Build history of the part. All positions in model axes, mm. A direction names the side the tool comes from. Coordinates: 2 decimals unless noted, no trailing zeros. Write each loop counter-clockwise with the first axis right and the second up, starting at its lowest first coordinate (ties: lowest second). Pieces come first, ordered by that corner, then holes. Notation, with made-up numbers: (-22, 52) -> (18, 52) arc R21 cw to (18, 80) -> close; hole circle Ø11 at (25, 1.5). An arc over 180 degrees is marked (long way). Write each question's results on one line, items separated by ' | '. Start each with the question number.
Q1. Saw through at B-B on x = 124. Give the cut face in (y, z), and give its area (3 significant figures).
Q2. Saw through at C-C on x = 42.5. Give the cut face in (y, z), and give its area (3 significant figures).
Q3. Drop flat-ended pins along their axis: pin 1 Ø9 at (x, y) = (-13, -40.5) entering from +Z; pin 2 Ø4 at (x, z) = (-7, -79) entering from -Y; pin 3 Ø15 at (x, y) = (-15.5, 48.5) entering from -Z. Give the stop position or say it passes through.
Q4. Tool access for faces 1 (the face through (-7, 0, 12.5)), 2 (the face through (0, -83, 57)), 3 (the face through (15.63, 63.375, 139.79)), 4 (the face through (-14.79, 21.125, 55.637)), 5 (the face through (84, -2, 125)): list every direction of +Z, -Z, +X, -X, +Y, -Y with a clear straight run to the whole face (end or side of a thin tool).
Q5. Saw through at D-D on z = 0. Give the cut face in (x, y).
Q6. Saw through at A-A on z = -128.5. Give the cut face in (x, y), and give its area (3 significant figures).
Q7. Two-plate mould, pull along Z, no slides. Class faces 6 (the face through (4, -77, 125)), 7 (the face through (79, -125, -2)), 8 (the face through (-8.963, 12.104, 55.638)): released by +Z, released by -Z, zero draft, split by the parting line, or undercut.
Q8. Drill centre lines: line 1 (Z direction, x = -2, y = 21); line 2 (Z direction, x = 32.5, y = 97); line 3 (X direction, y = 23.5, z = 77.5). Where is each one in solid material? Low to high.
from build123d import *

# Parameters (mm, degrees)
IZIM1_W                          = 250
IZIM1_H                          = 250
Y_KSEKLIK_EKSTR_ZYON1_DEPTH      = 150
IZIM2_R                          = 108.43509044
KES_EKSTR_ZYON1_DEPTH            = 60
KES_EKSTR_ZYON1_TAPER            = 60
IZIM3_W                          = 25
IZIM3_H                          = 250
Y_KSEKLIK_EKSTR_ZYON2_DEPTH      = 30
Y_KSEKLIK_EKSTR_ZYON3_DEPTH      = 30
Y_KSEKLIK_EKSTR_ZYON3_DEPTH_BACK = 280


with BuildPart() as part:
    # Çizim1 → Yükseklik-Ekstrüzyon1 (new body)
    with BuildSketch(Plane(origin=(0, 0, 0), x_dir=(0, 0, -1), z_dir=(1, 0, 0))):
        Rectangle(IZIM1_W, IZIM1_H)
    extrude(amount=Y_KSEKLIK_EKSTR_ZYON1_DEPTH)

    # Çizim2 → Kes-Ekstrüzyon1 (cut)
    with BuildSketch(Plane(origin=(150, 0, 0), x_dir=(0, 0, -1), z_dir=(1, 0, 0))):
        Circle(IZIM2_R)
    extrude(amount=-KES_EKSTR_ZYON1_DEPTH, taper=KES_EKSTR_ZYON1_TAPER, mode=Mode.SUBTRACT)

    # Çizim3 → Yükseklik-Ekstrüzyon2 (add)
    with BuildSketch(Plane.ZY):
        with Locations((-112.5, 0)):
            Rectangle(IZIM3_W, IZIM3_H)
        with Locations((112.5, 0)):
            Rectangle(IZIM3_W, IZIM3_H)
        Rectangle(IZIM3_W, IZIM3_H)
    extrude(amount=Y_KSEKLIK_EKSTR_ZYON2_DEPTH)

    # Çizim4 → Yükseklik-Ekstrüzyon3 (add, two sides: drawn at the far end of the back side and taken through both)
    with BuildSketch(Plane.XY.offset(125).offset(-Y_KSEKLIK_EKSTR_ZYON3_DEPTH_BACK)):
        Polygon((60, 125), (-30, 0), (60, -125), (73.958390673, -125), (68.115343415, -119.156952742), (-17.677662559, 0), (68.115343415, 119.156952742), (72.322337441, 125), align=None)
    extrude(amount=Y_KSEKLIK_EKSTR_ZYON3_DEPTH + Y_KSEKLIK_EKSTR_ZYON3_DEPTH_BACK)


solid = part.part
Returned:
1) outline: (-125, -125) -> (125, -125) -> (125, 125) -> (-125, 125) -> close; hole circle Ø126.8 at (0, 0) | area: 49,900 mm2
2) outline: (-125, -125) -> (-100.69, -125) -> (-100.69, -155) -> (-83.58, -155) -> (-83.58, -125) -> (83.58, -125) -> (83.58, -155) -> (100.69, -155) -> (100.69, -125) -> (125, -125) -> (125, 125) -> (100.69, 125) -> (100.69, 155) -> (83.58, 155) -> (83.58, 125) -> (-83.58, 125) -> (-83.58, 155) -> (-100.69, 155) -> (-100.69, 125) -> (-125, 125) -> close | area: 64,600 mm2
3) pin 1: stops at z = 125 | pin 2: stops at y = -34.72 | pin 3: stops at z = -125
4) face 1: none | face 2: -X, -Y | face 3: +Z, -X, +Y | face 4: -X, +Y | face 5: +Z, +X
5) outline: (-30, -125) -> (150, -125) -> (150, -108.44) -> (90, -4.51) -> (90, 4.51) -> (150, 108.44) -> (150, 125) -> (-30, 125) -> close
6) outline: (-30, 0) -> (60, -125) -> (73.96, -125) -> (68.12, -119.16) -> (-17.68, 0) -> (72.32, 125) -> (60, 125) -> close | area: 3,090 mm2
7) face 6: released by +Z | face 7: zero draft | face 8: undercut
8) line 1: z = -125 to -100, -12.5 to 12.5, 100 to 125 | line 2: z = -125 to 125 | line 3: x = -13.08 to -0.76, 0 to 134.15
